For this review, use the dimensioned drawing (mm, ordinates from the lowest corner) and the shaded views. A direction names the side the tool comes from. Coordinates: 2 decimals unless noted, no trailing zeros. Order: outer loops, then holes, each group sorted by start corner. A loop starts at its lowest first (then second) coordinate and runs counter-clockwise, first axis right, second up. Notation, with made-up numbers: (-2, 78.25) -> (52, 78.25) arc R24 ccw to (52, 98.25) -> close; hole circle Ø7 at (41.25, 19). An arc over 180 degrees is marked (long way). Return JSON: item names as keys, results as strings. Group by question number.
Item 1: Take a section at C-C (z = 6.5). Count the separate pieces of the cut face and the enclosed holes in it, then the cut area to 3 significant figures.
Item 2: Insertion check: pin 1 (2 mm diameter, centred on x = 85.5, z = 3, fed in from -Y); pin 2 (3 mm diameter, centred on x = 97, y = 116.5, fed in from -Z). Each pin has a flat end and moves straight along its axis. Give the tip position at first contact, or say it passes through.
Item 3: Machinability: for the marked faces 1, 2 and 3, which of the approach directions +Z, -Z, +X, -X, +Y, -Y give a long, thin tool a straight path to every point of the face, cutting with its end or side? Answer none if there is none.
Item 4: Take a section at A-A (x = 54.9). Write out the cut boundary in (y, z).
Item 5: Draft analysis for pull direction X (two halves, no side actions). For the marked faces 4, 5 and 6, state which applies: +X half, -X half, draft (parallel to the pull), parting line (faces both ways), or undercut.
Item 6: Take a section at B-B (y = 87.7). Write out the cut boundary in (x, z), then the cut area to 3 significant figures.
Item 7: For line 1 along X through (y, z) = (27, 7.5); line 2 along X through (y, z) = (51.5, 7.75) (1 decimal); line 3 along Y through (x, z) = (54.9, 4.25), list the stretches that pass through material, from the lowest coordinate up.
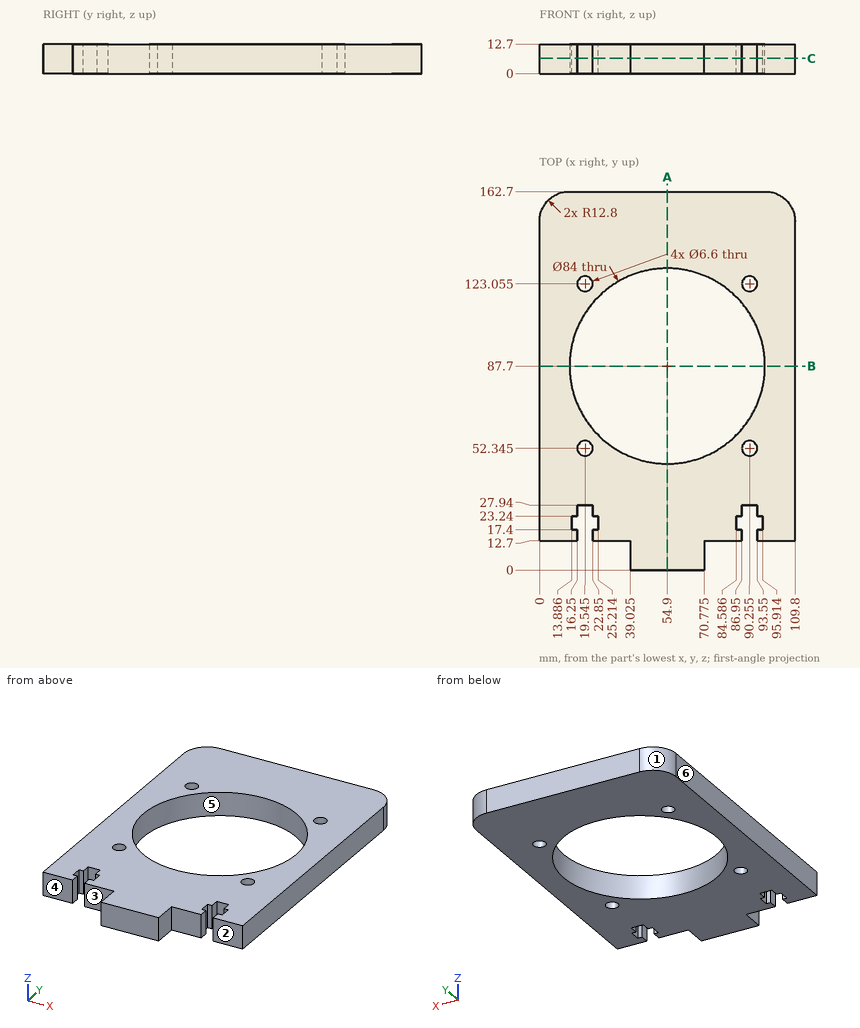
Findings below:
{
 "1": {"separate pieces": "1", "enclosed holes": "5", "area": "10,900 mm2"},
 "2": {"pin 1": "stops at y = 12.7", "pin 2": "stops at z = 0"},
 "3": {"face 1": "+Z, -Z, -X, +Y", "face 2": "+Z, -Z, +X, -Y", "face 3": "+Z, -Z, -X, -Y"},
 "4": {"outline": "(0, 0) -> (45.7, 0) -> (45.7, 12.7) -> (0, 12.7) -> close; (129.7, 0) -> (162.7, 0) -> (162.7, 12.7) -> (129.7, 12.7) -> close"},
 "5": {"face 4": "draft", "face 5": "undercut", "face 6": "-X half"},
 "6": {"outline": "(0, 0) -> (12.9, 0) -> (12.9, 12.7) -> (0, 12.7) -> close; (96.9, 0) -> (109.8, 0) -> (109.8, 12.7) -> (96.9, 12.7) -> close", "area": "328 mm2"},
 "7": {"line 1": "x = 0 to 16.25, 22.85 to 86.95, 93.55 to 109.8", "line 2": "x = 0 to 16.4, 22.7 to 33.6, 76.2 to 87.1, 93.4 to 109.8", "line 3": "y = 0 to 45.7, 129.7 to 162.7"}
}
